The model under review builds one solid part; all positions refer to its coordinate system, in mm. Coordinates: 2 decimals unless noted, no trailing zeros. Loops run counter-clockwise (first coordinate to the right, second up) from the corner with the lowest first, then second, coordinate; pieces in that order, holes last. Notation, with made-up numbers: M -9.5,1.5 L 41.5,1.5 A22 ccw 41.5,26.5 Z; hole C 30.5,42.5 d3. An arc over 180 degrees is marked long. Use CSV: the item, a comma, the result in double quotes. Start each with the question number.
from build123d import *

# Parameters (mm, degrees)
BOSS_EXTRU_2_DEPTH      = 73
ESQUISSE6_W             = 6
ESQUISSE6_H             = 5
ENL_V_MAT_EXTRU_3_DEPTH = 83.675570757
ESQUISSE7_R             = 1.75
ENL_V_MAT_EXTRU_4_DEPTH = 12
ENL_V_START             = -12
ESQUISSE8_R             = 1.75
ENL_V_MAT_EXTRU_5_DEPTH = 12
CONG_1_R                = 3
ENL_V_START_2           = -3
ENL_V_MAT_EXTRU_6_DEPTH = 2.6
ENL_V_START_3           = -5.6
ENL_V_MAT_EXTRU_7_DEPTH = 2.6
CHANFREIN1_SIZE         = 1.154700538
CHANFREIN1_SIZE_2       = 2


with BuildPart() as part:
    # Esquisse3 → Boss.-Extru.2 (new body)
    with BuildSketch(Plane.XY):
        with BuildLine():
            ThreePointArc((-5, 37.165171868), (0, 37.5), (5, 37.165171868))
            Line((5, 37.165171868), (5, 30.214079913))
            Line((5, 30.214079913), (-5, 30.214079913))
            Line((-5, 30.214079913), (-5, 37.165171868))
        make_face()
    extrude(amount=BOSS_EXTRU_2_DEPTH)

    # Esquisse6 → Enlèv. mat.-Extru.3 (cut, through all)
    with BuildSketch(Plane.ZY.offset(5)):
        with Locations((20, 37.714079913)):
            Rectangle(ESQUISSE6_W, ESQUISSE6_H)
        with Locations((53, 37.714079913)):
            Rectangle(ESQUISSE6_W, ESQUISSE6_H)
    extrude(amount=-ENL_V_MAT_EXTRU_3_DEPTH, mode=Mode.SUBTRACT)

    # Esquisse7 → Enlèv. mat.-Extru.4 (cut)
    with BuildSketch(Plane.XY.offset(73)):
        with Locations((0, 33.75)):
            Circle(ESQUISSE7_R)
    extrude(amount=-ENL_V_MAT_EXTRU_4_DEPTH, mode=Mode.SUBTRACT)

    # Esquisse8 → Enlèv. mat.-Extru.5 (cut)
    with BuildSketch(Plane(origin=(0, 0, 0), x_dir=(-1, 0, 0), z_dir=(0, 0, -1)).offset(ENL_V_START)):
        with Locations(Location((0, 33.75, 0), (0, 0, 180))):
            Circle(ESQUISSE8_R)
    extrude(amount=ENL_V_MAT_EXTRU_5_DEPTH, mode=Mode.SUBTRACT)

    # Congé1
    cong_1_edges = [part.edges().sort_by_distance(p)[0] for p in [
        (5, 35.214079913, 20),
        (-5, 35.214079913, 20),
        (5, 35.214079913, 53),
        (-5, 35.214079913, 53),
    ]]
    fillet(cong_1_edges, radius=CONG_1_R)

    # Esquisse9 → Enlèv. mat.-Extru.6 (cut)
    with BuildSketch(Plane(origin=(0, 0, 0), x_dir=(-1, 0, 0), z_dir=(0, 0, -1)).offset(ENL_V_START_2)):
        with BuildLine():
            Line((-2.85, 37.391543162), (-2.85, 31.995448267))
            Line((-2.85, 31.995448267), (0, 30.35))
            Line((0, 30.35), (2.85, 31.995448267))
            Line((2.85, 31.995448267), (2.85, 37.391543162))
            ThreePointArc((2.85, 37.391543162), (0, 37.5), (-2.85, 37.391543162))
        make_face()
    extrude(amount=-ENL_V_MAT_EXTRU_6_DEPTH, mode=Mode.SUBTRACT)

    # Esquisse10 → Enlèv. mat.-Extru.7 (cut)
    with BuildSketch(Plane.XY.offset(73).offset(ENL_V_START_3)):
        with BuildLine():
            Line((-2.85, 37.391543162), (-2.85, 31.995448267))
            Line((-2.85, 31.995448267), (0, 30.35))
            Line((0, 30.35), (2.85, 31.995448267))
            Line((2.85, 31.995448267), (2.85, 37.391543162))
            ThreePointArc((2.85, 37.391543162), (0, 37.5), (-2.85, 37.391543162))
        make_face()
    extrude(amount=ENL_V_MAT_EXTRU_7_DEPTH, mode=Mode.SUBTRACT)

    # Chanfrein1
    # the kernel refuses this chamfer: 2, 1.154700538 mm, written as the material it takes off along each edge
    with BuildSketch(Plane(origin=(5, 30.214079913, -5.174171509), x_dir=(0.0578938624026711, 0.9983227437537925, 0), z_dir=(0, 0, 1)), Plane(origin=(-5, 30.214079913, -5.174171509), x_dir=(0.9983227437537925, -0.05789386240267115, 0), z_dir=(0, 0, 1))) as chanfrein1_piece_1:
        Polygon((CHANFREIN1_SIZE * 0.998322744082, CHANFREIN1_SIZE * 0.0578938624217), (-CHANFREIN1_SIZE_2 * 0.0578938624027, CHANFREIN1_SIZE_2 * 0.998322743754), (0, 0), align=None)
    extrude(amount=83.348343019, mode=Mode.SUBTRACT)


solid = part.part
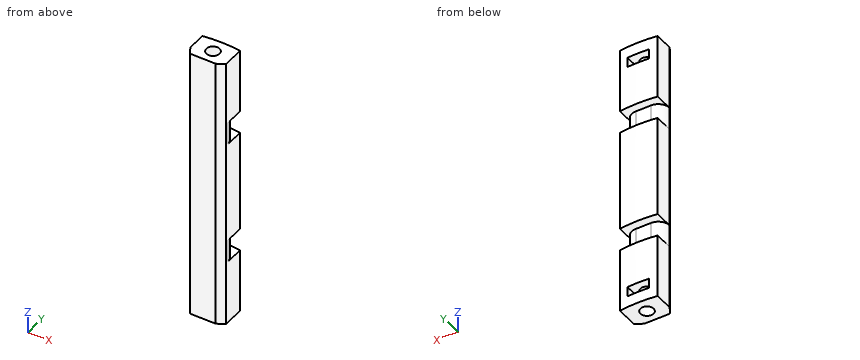
1. Insertion check: pin 1 Ø3 at (x, z) = (1, 20.5) entering from +Y; pin 2 Ø1.7 at (x, y) = (0.5, 34) entering from -Z; pin 3 Ø6 at (x, z) = (2, 20.5) entering from +Y; pin 4 Ø2.5 at (x, y) = (2, 35.5) entering from -Z. Each pin has a flat end and moves straight along its axis. Give the tip position at first contact, or say it passes through.
2. To check wall thickness, follow line 1 along Z through (x, y) = (3.75, 36); line 2 along Z through (x, y) = (-2.25, 34); line 3 along Z through (x, y) = (1, 35.75). State the ranges of each line that lie inside material, in increasing order.
3. Add section B-B (x = 0.75). Give the number of separate pieces and of enclosed holes in the cut face, plus the area to 3 significant figures.
4. Add section A-A (z = 21). Write out the cut boundary in (x, y).
5. Add section C-C (z = 13). Write out the cut boundary in (x, y), plus the area to 3 significant figures.
Solved:
1,pin 1,"stops at y = 35.21"
1,pin 2,"stops at z = 12"
1,pin 3,"stops at y = 37.5"
1,pin 4,"stops at z = 0"
2,line 1,"z = 0 to 17, 23 to 50, 56 to 73"
2,line 2,"z = 0 to 3, 5.6 to 67.4, 70 to 73"
2,line 3,"z = 0 to 3, 5.6 to 17, 23 to 50, 56 to 67.4, 70 to 73"
3,separate pieces,"3"
3,enclosed holes,"0"
3,area,"410 mm^2"
4,outline,"M -5,32.21 L -3.85,30.21 L 3,30.21 L 5,31.37 L 5,32.21 A3 ccw 2,35.21 L -2,35.21 A3 ccw Z"
5,outline,"M -5,32.21 L -3.85,30.21 L 3,30.21 L 5,31.37 L 5,37.17 A37.5 ccw -5,37.17 Z"
5,area,"69.4 mm^2"
